from build123d import *

# Parameters (mm, degrees)
SKETCH1_W           = 200
SKETCH1_H           = 8
BOSS_EXTRUDE1_DEPTH = 0.4
SKETCH2_W           = 3
SKETCH2_H           = 3
BOSS_EXTRUDE2_DEPTH = 1.75
SKETCH3_R           = 0.95
CUT_EXTRUDE1_DEPTH  = 0.1
LPATTERN1_COUNT     = 12
LPATTERN1_PITCH     = 16.5
SKETCH4_W           = 1.6
SKETCH4_H           = 4
BOSS_EXTRUDE3_DEPTH = 1
LPATTERN2_COUNT     = 4
LPATTERN2_PITCH     = 49.1


with BuildPart() as part:
    # Sketch1 → Boss-Extrude1 (new body)
    with BuildSketch(Plane(origin=(0, 0, 0), x_dir=(1, 0, 0), z_dir=(0, 1, 0))):
        Rectangle(SKETCH1_W, SKETCH1_H)
    extrude(amount=BOSS_EXTRUDE1_DEPTH)

    # Sketch2 → Boss-Extrude2 (add)
    with BuildSketch(Plane(origin=(0, 0.4, 0), x_dir=(1, 0, 0), z_dir=(0, 1, 0))):
        with Locations((91.9, 0)):
            Rectangle(SKETCH2_W, SKETCH2_H)
    boss_extrude2 = extrude(amount=BOSS_EXTRUDE2_DEPTH)

    # Sketch3 → Cut-Extrude1 (cut)
    with BuildSketch(Plane(origin=(0, 2.15, 0), x_dir=(1, 0, 0), z_dir=(0, 1, 0))):
        with Locations(Location((91.9, 0, 0), (0, 0, 270))):
            Circle(SKETCH3_R)
    cut_extrude1 = extrude(amount=-CUT_EXTRUDE1_DEPTH, mode=Mode.SUBTRACT)

    # LPattern1: Boss-Extrude2, Cut-Extrude1 ×12
    with Locations(*[(-i * LPATTERN1_PITCH, 0, 0) for i in range(1, LPATTERN1_COUNT)]):
        add(boss_extrude2)
        add(cut_extrude1, mode=Mode.SUBTRACT)

    # Sketch4 → Boss-Extrude3 (add)
    with BuildSketch(Plane(origin=(0, 0.4, 0), x_dir=(1, 0, 0), z_dir=(0, 1, 0))):
        with Locations((67.4, 0)):
            Rectangle(SKETCH4_W, SKETCH4_H)
    boss_extrude3 = extrude(amount=BOSS_EXTRUDE3_DEPTH)

    # LPattern2: Boss-Extrude3 ×4
    with Locations(*[(-i * LPATTERN2_PITCH, 0, 0) for i in range(1, LPATTERN2_COUNT)]):
        add(boss_extrude3)


solid = part.part
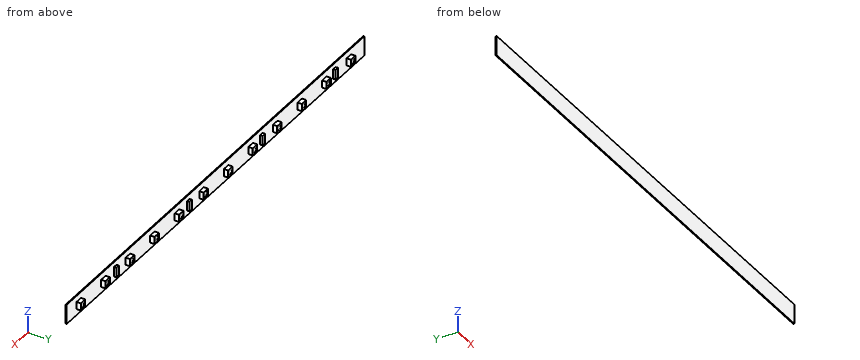
For this review, take the finished solid that the model builds, in its own axes (mm). Round coordinates to 2 decimals unless told otherwise and drop trailing zeros. Loops run counter-clockwise (first coordinate to the right, second up) from the corner with the lowest first, then second, coordinate; pieces in that order, holes last. Notation, with made-up numbers: (20, 41.25) - (64, 41.25) arc R22 cw to (64, 49.25) - close; hole circle Ø2 at (-13, -35.5). An arc over 180 degrees is marked (long way). Put each result on its own line as item: value. Start each with the question number.
1. For probe 1 along X at (y, z) = (0.9, 1.75); probe 2 along Z at (x, y) = (75.4, 2.1); probe 3 along Y at (x, z) = (-76, 1.75), list the stretches that pass through material, from the lowest coordinate up. Write a range as [from, to].
2. Consider section A-A on y = 0.9. State how many separate pieces and enclosed holes the cut face has, plus the area to 3 significant figures.
3. Insertion check: P1, Ø1.5, axis at x = -73.1, z = 0, coming from the +Y side; P2, Ø0.5, axis at x = -80, y = 1, coming from the -Z side; P3, Ø0.9, axis at y = 1.5, z = -0.5, coming from the +X side. Each pin has a flat end and moves straight along its axis. Give the tip position at first contact, or say it passes through.
4. Consider section B-B on x = 53. State the section outline as (y, z) points, plus the area to 3 significant figures.
Result sheet:
1. probe 1: [-80.7, -79.1], [-31.6, -30], [17.5, 19.1], [66.6, 68.2]
1. probe 2: [-1.5, -0.95], [0.95, 1.5]
1. probe 3: [0, 0.4]
2. separate pieces: 16
2. enclosed holes: 0
2. area: 134 mm^2
3. P1: y = 2.05
3. P2: z = -2
3. P3: x = 93.4
4. outline: (0, -4) - (0.4, -4) - (0.4, 4) - (0, 4) - close
4. area: 3.20 mm^2
